Read the model definition and answer for the solid it produces. Units are mm, in the model's axes. Face numbers are marked on the shaded views. Give positions to 0.01 mm unless a question says otherwise; leave off trailing zeros. Write each loop counter-clockwise with the first axis right and the second up, starting at its lowest first coordinate (ties: lowest second). Pieces come first, ordered by that corner, then holes. Notation, with made-up numbers: M 44,-26 L 62,-26 A17 cw 62,-11 Z; hole C 33,74.5 d4. An arc over 180 degrees is marked long. Use a Markdown table: item, result. Add a question column.
Item 1: A cutting plane is placed at D-D on z = 23. Determine the outline of the cut face in (x, y), then the cut area to 3 significant figures.
Item 2: Given P1, Ø1.7, axis at x = -17, z = 9.5, coming from the +Y side; P2, Ø2, axis at y = 0, z = 10, coming from the +X side; P3, Ø1, axis at x = 17.5, z = 10.5, coming from the -Y side; P4, Ø1, axis at x = 17, y = 1.5, coming from the -Z side, each flat-ended and moving along its own axis, determine where each tip first touches the part or whether it passes through.
Item 3: A cutting plane is placed at C-C on z = 6.5. Determine the outline of the cut face in (x, y).
Item 4: A cutting plane is placed at A-A on z = 34. Determine the outline of the cut face in (x, y).
Item 5: A cutting plane is placed at B-B on x = 0. Determine the outline of the cut face in (y, z), then the cut area to 3 significant figures.
Item 6: The mould has two halves that part along X. Classify the marked faces 1, 2, 3 and 4: pulls with the +X half, pulls with the -X half, needs draft (parallel to the pull), parting line crosses it, or undercut.
Item 7: Consider probe 1 along Y at (x, z) = (0, 23.5); probe 2 along X at (y, z) = (0, 36.5); probe 3 along X at (y, z) = (17, 20.5). Determine where each line is inside the solid, lowest interval first. Write a range as [from, to].
from build123d import *

# Parameters (mm, degrees)
SKETCH2_W           = 46.2
SKETCH2_H           = 38
SKETCH2_R           = 13.3
BOSS_EXTRUDE1_DEPTH = 48.5
SKETCH3_R           = 1.7
CUT_EXTRUDE1_DEPTH  = 70.625354577
SKETCH4_W           = 3.4
SKETCH4_H           = 7
CUT_EXTRUDE2_DEPTH  = 16
CUT_EXTRUDE3_DEPTH  = 15.5
CUT_EXTRUDE4_DEPTH  = 45.537736882
FILLET1_R           = 10
CHAMFER1_SIZE       = 1.6
CHAMFER2_SIZE       = 1.6
CHAMFER3_SIZE       = 1.6
CHAMFER4_SIZE       = 1.6


with BuildPart() as part:
    # Sketch2 → Boss-Extrude1 (new body)
    with BuildSketch(Plane.XY):
        Rectangle(SKETCH2_W, SKETCH2_H)
        with Locations(Location((0, 0, 0), (0, 0, 180))):
            Circle(SKETCH2_R, mode=Mode.SUBTRACT)
    extrude(amount=BOSS_EXTRUDE1_DEPTH)

    # Sketch3 → Cut-Extrude1 (cut, through all)
    with BuildSketch(Plane(origin=(23.1, 0, 0), x_dir=(0, 0, -1), z_dir=(1, 0, 0))):
        with Locations((-10, 0)):
            Circle(SKETCH3_R)
    extrude(amount=-CUT_EXTRUDE1_DEPTH, mode=Mode.SUBTRACT)

    # Sketch4 → Cut-Extrude2 (cut)
    with BuildSketch(Plane(origin=(0, 0, 0), x_dir=(-1, 0, 0), z_dir=(0, 0, -1))):
        with Locations((-17.4, 0)):
            Rectangle(SKETCH4_W, SKETCH4_H)
        with Locations((17.4, 0)):
            Rectangle(SKETCH4_W, SKETCH4_H)
    extrude(amount=-CUT_EXTRUDE2_DEPTH, mode=Mode.SUBTRACT)

    # Sketch1 → Cut-Revolve1 (revolve, cut)
    with BuildSketch(Plane(origin=(0, 0, 0), x_dir=(0, 0, -1), z_dir=(1, 0, 0)), mode=Mode.PRIVATE) as cut_revolve1_sk:
        Polygon((0, 0), (0, 13.3), (-33, 13.3), (-33, 15), (-48.5, 15), (-48.5, 0), align=None)
    revolve(cut_revolve1_sk.sketch.rotate(Axis((0, 0, 1000), (0, 0, -1)), 90), axis=Axis((0, 0, 1000), (0, 0, -1)), mode=Mode.SUBTRACT)

    # Sketch5 → Cut-Extrude3 (cut)
    with BuildSketch(Plane.XY.offset(48.5)):
        Polygon((12.638406773, 10.39522635), (11.06006345, 10.132867141), (12.076444851, 8.897161332), align=None)
    extrude(amount=-CUT_EXTRUDE3_DEPTH, mode=Mode.SUBTRACT)

    # Sketch6 → Cut-Extrude4 (cut, through all)
    with BuildSketch(Plane.XY.offset(33)):
        Polygon((11.32335828, 9.313584733), (9.745014957, 9.051225524), (10.761396359, 7.815519715), align=None)
    extrude(amount=-CUT_EXTRUDE4_DEPTH, mode=Mode.SUBTRACT)

    # Fillet1
    fillet1_edges = [part.edges().sort_by_distance(p)[0] for p in [
        (23.1, -19, 24.25),
        (-23.1, -19, 24.25),
        (-23.1, 19, 24.25),
        (23.1, 19, 24.25),
    ]]
    fillet(fillet1_edges, radius=FILLET1_R)

    # Chamfer1
    chamfer1_edges = [part.edges().sort_by_distance(p)[0] for p in [
        (0, 19, 48.5),
        (-23.1, 0, 48.5),
        (20.171067812, 16.071067812, 48.5),
        (-20.171067812, 16.071067812, 48.5),
        (-20.171067812, -16.071067812, 48.5),
        (20.171067812, -16.071067812, 48.5),
        (23.1, 0, 48.5),
        (0, -19, 48.5),
    ]]
    chamfer(chamfer1_edges, length=CHAMFER1_SIZE)

    # Chamfer2
    # the kernel refuses this chamfer: 1.6 mm, written as the material it takes off along each edge
    with BuildSketch(Plane(origin=(0, 0, 33), x_dir=(-1, 0, 0), z_dir=(0, 1, 0))) as chamfer2_piece_1:
        Polygon((13.3, -CHAMFER2_SIZE), (13.3 + CHAMFER2_SIZE, 0), (13.3, 0), align=None)
    revolve(axis=Axis((0, 0, 33), (0, 0, 1)), revolution_arc=233.756192623, mode=Mode.SUBTRACT)
    with BuildSketch(Plane(origin=(0, 0, 33), x_dir=(0.905245194595796, 0.42488955936951367, 0), z_dir=(0.42488955936951367, -0.905245194595796, 0))) as chamfer2_piece_2:
        Polygon((13.3, -CHAMFER2_SIZE), (13.3 + CHAMFER2_SIZE, 0), (13.3, 0), align=None)
    revolve(axis=Axis((0, 0, 33), (0, 0, 1)), revolution_arc=154.856326918, mode=Mode.SUBTRACT)

    # Chamfer3
    chamfer3_edges = [part.edges().sort_by_distance(p)[0] for p in [
        (15.7, 0, 0),
        (17.4, 3.5, 0),
        (19.1, 0, 0),
        (17.4, -3.5, 0),
        (-17.4, -3.5, 0),
        (-19.1, 0, 0),
        (-17.4, 3.5, 0),
        (-15.7, 0, 0),
    ]]
    chamfer(chamfer3_edges, length=CHAMFER3_SIZE)

    # Chamfer4
    chamfer4_edges = [part.edges().sort_by_distance(p)[0] for p in [
        (23.1, 0, 0),
        (0, -19, 0),
        (-23.1, 0, 0),
        (0, 19, 0),
        (20.171067812, 16.071067812, 0),
        (-20.171067812, 16.071067812, 0),
        (-20.171067812, -16.071067812, 0),
        (20.171067812, -16.071067812, 0),
    ]]
    chamfer(chamfer4_edges, length=CHAMFER4_SIZE)


solid = part.part
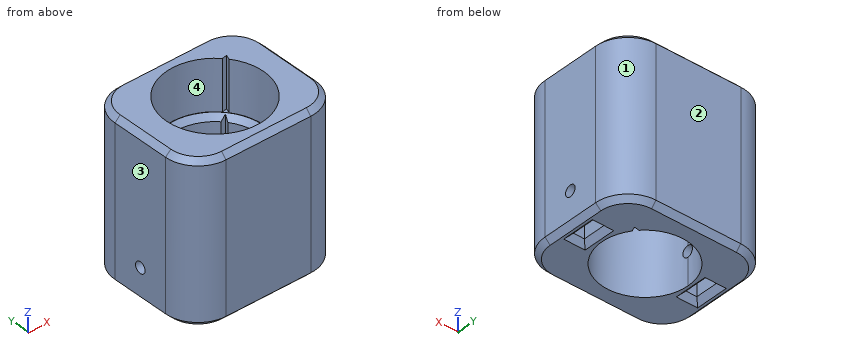
Filled in:
| question | item | result |
|---|---|---|
| 1 | outline | M -23.1,-9 A10 ccw -13.1,-19 L 13.1,-19 A10 ccw 23.1,-9 L 23.1,9 A10 ccw 13.1,19 L -13.1,19 A10 ccw -23.1,9 Z; hole M 9.75,9.05 A13.3 ccw long 10.76,7.82 L 11.32,9.31 Z |
| 1 | area | 1,110 mm² |
| 2 | P1 | y = 18.52 |
| 2 | P2 | through |
| 2 | P3 | y = -18.21 |
| 2 | P4 | z = 16 |
| 3 | outline | M -23.1,-9 A10 ccw -13.1,-19 L 13.1,-19 A10 ccw 23.1,-9 L 23.1,9 A10 ccw 13.1,19 L -13.1,19 A10 ccw -23.1,9 Z; hole M -19.1,-3.5 L -15.7,-3.5 L -15.7,3.5 L -19.1,3.5 Z; hole M 9.75,9.05 A13.3 ccw long 10.76,7.82 L 11.32,9.31 Z; hole M 15.7,-3.5 L 19.1,-3.5 L 19.1,3.5 L 15.7,3.5 Z |
| 4 | outline | M -23.1,-9 A10 ccw -13.1,-19 L 13.1,-19 A10 ccw 23.1,-9 L 23.1,9 A10 ccw 13.1,19 L -13.1,19 A10 ccw -23.1,9 Z; hole M 11.06,10.13 A15 ccw long 12.08,8.9 L 12.64,10.4 Z |
| 5 | outline | M -19,1.6 L -17.4,0 L -13.3,0 L -13.3,31.4 L -14.9,33 L -15,33 L -15,48.5 L -17.4,48.5 L -19,46.9 Z; M 13.3,0 L 17.4,0 L 19,1.6 L 19,46.9 L 17.4,48.5 L 15,48.5 L 15,33 L 14.9,33 L 13.3,31.4 Z |
| 5 | area | 493 mm² |
| 6 | face 1 | pulls with the +X half |
| 6 | face 2 | needs draft |
| 6 | face 3 | pulls with the -X half |
| 6 | face 4 | undercut |
| 7 | probe 1 | [-19, -13.3], [13.3, 19] |
| 7 | probe 2 | [-23.1, -15], [15, 23.1] |
| 7 | probe 3 | [-19.1, 19.1] |
